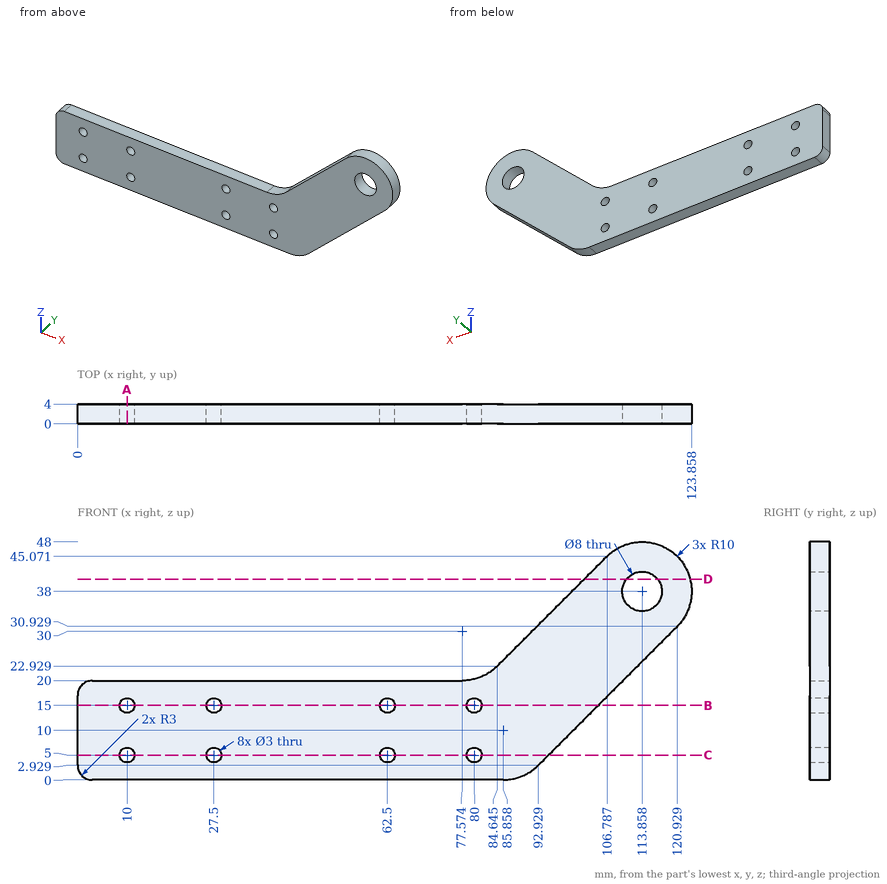
Geometry: see drawing. Coordinates: mm, zero at the bounding-box minimum. Give positions to 0.01 mm unless a question says otherwise; leave off trailing zeros. Loops run counter-clockwise (first coordinate to the right, second up) from the corner with the lowest first, then second, coordinate; pieces in that order, holes last. Notation, with made-up numbers: (-7.75, 87) -> (18.25, 87) arc R23 cw to (18.25, 114) -> close; hole circle Ø8 at (58, 78). An arc over 180 degrees is marked (long way). Use one line per item in the form item = value.
Item 1: Section query C-C on z = 5. Output: boundary loops of the cut face in (x, y), and give its area (3 significant figures).
A:
outline = (0, 0) -> (8.5, 0) -> (8.5, 4) -> (0, 4) -> close; (11.5, 0) -> (26, 0) -> (26, 4) -> (11.5, 4) -> close; (29, 0) -> (61, 0) -> (61, 4) -> (29, 4) -> close; (64, 0) -> (78.5, 0) -> (78.5, 4) -> (64, 4) -> close; (81.5, 0) -> (95, 0) -> (95, 4) -> (81.5, 4) -> close
area = 332 mm^2
Item 2: Section query B-B on z = 15. Output: boundary loops of the cut face in (x, y).
A:
outline = (0, 0) -> (8.5, 0) -> (8.5, 4) -> (0, 4) -> close; (11.5, 0) -> (26, 0) -> (26, 4) -> (11.5, 4) -> close; (29, 0) -> (61, 0) -> (61, 4) -> (29, 4) -> close; (64, 0) -> (78.5, 0) -> (78.5, 4) -> (64, 4) -> close; (81.5, 0) -> (105, 0) -> (105, 4) -> (81.5, 4) -> close
Item 3: Line query: probe 1 along X at (y, z) = (1.85, 5); probe 2 along Z at (x, y) = (80, 3.15); probe 3 along Z at (x, y) = (79.5, 2.8) (1 decimal). Output: solid intervals per line, ascending.
A:
probe_1 = 0 to 8.5, 11.5 to 26, 29 to 61, 64 to 78.5, 81.5 to 95
probe_2 = 0 to 3.5, 6.5 to 13.5, 16.5 to 20.3
probe_3 = 0 to 3.6, 6.4 to 13.6, 16.4 to 20.2
Item 4: Section query A-A on x = 10. Output: boundary loops of the cut face in (y, z).
A:
outline = (0, 0) -> (4, 0) -> (4, 3.5) -> (0, 3.5) -> close; (0, 6.5) -> (4, 6.5) -> (4, 13.5) -> (0, 13.5) -> close; (0, 16.5) -> (4, 16.5) -> (4, 20) -> (0, 20) -> close
Item 5: Pin query (flat end, axial travel): P1, Ø2, axis at x = 23.5, y = 1, coming from the +Z side. Return the tip coordinate at first contact, or that it passes through.
A:
P1 = 20
Item 6: Section query D-D on z = 40.5. Output: boundary loops of the cut face in (x, y) (1 decimal).
A:
outline = (102.2, 0) -> (110.7, 0) -> (110.7, 4) -> (102.2, 4) -> close; (117, 0) -> (123.5, 0) -> (123.5, 4) -> (117, 4) -> close
